from build123d import *

# Parameters (mm, degrees)
F0_R     = 1.55
F0_R_2   = 2.05
F0_R_3   = 11
F1_DEPTH = 4


with BuildPart() as f1:
    # F0 (on Front) → F1 (new body)
    with BuildSketch(Plane.XZ):
        with BuildLine():
            Line((-12.9276869952, -14.7702103927), (49.2744245402, -25.0594563055))
            ThreePointArc((49.2744245402, -25.0594563055), (61.2632923167, -19.4743843221), (57.2253318853, -6.8799071524))
            Line((57.2253318853, -6.8799071524), (-12.5790872929, 34.7723583687))
            Line((-12.5790872929, 34.7723583687), (-35.6180453168, 48.5196942571))
            ThreePointArc((-35.6180453168, 48.5196942571), (-39.3883061053, 49.0778177624), (-42.4565310048, 46.8167639757))
            Line((-42.4565310048, 46.8167639757), (-44.283169795, 43.8016410413))
            Line((-44.283169795, 43.8016410413), (-68.4894634868, 3.7363676474))
            ThreePointArc((-68.4894634868, 3.7363676474), (-69.1796280017, 0.6014549382), (-67.8214663387, -2.3070501159))
            Line((-67.8214663387, -2.3070501159), (-54.0816127895, -16.6578253643))
            ThreePointArc((-54.0816127895, -16.6578253643), (-52.4335683043, -17.7983223484), (-50.4700412586, -18.200000748))
            Line((-50.4700412586, -18.200000748), (-21.8383905306, -18.200000748))
            ThreePointArc((-21.8383905306, -18.200000748), (-20.3097897038, -17.960607801), (-18.9275633798, -17.265352553))
            Line((-18.9275633798, -17.265352553), (-16.6545073746, -15.6378247392))
            ThreePointArc((-16.6545073746, -15.6378247392), (-14.877378135, -14.8333994398), (-12.9276869952, -14.7702103927))
        make_face()
        with BuildLine():
            ThreePointArc((-46.4896173713, 5.2461908635), (-45.1396173713, 6.5961908635), (-43.7896173713, 5.2461908635))
            Line((-43.7896173713, 5.2461908635), (-43.7896173713, -12.7538091365))
            ThreePointArc((-43.7896173713, -12.7538091365), (-45.1396173713, -14.1038091365), (-46.4896173713, -12.7538091365))
            Line((-46.4896173713, -12.7538091365), (-46.4896173713, 5.2461908635))
        make_face(mode=Mode.SUBTRACT)
        with BuildLine():
            Line((-41.1896173713, -13.2911801338), (-41.1896173713, 5.2461908635))
            ThreePointArc((-41.1896173713, 5.2461908635), (-38.1396173713, 8.2961908635), (-35.0896173713, 5.2461908635))
            Line((-35.0896173713, 5.2461908635), (-35.0896173713, -13.2911801338))
            ThreePointArc((-35.0896173713, -13.2911801338), (-38.1396173713, -16.3411801338), (-41.1896173713, -13.2911801338))
        make_face(mode=Mode.SUBTRACT)
        with Locations((-58.3313559954, 8.044780269)):
            Circle(F0_R, mode=Mode.SUBTRACT)
        with BuildLine():
            Line((-32.4896173713, -12.7538091365), (-32.4896173713, 5.2461908635))
            ThreePointArc((-32.4896173713, 5.2461908635), (-31.1396173713, 6.5961908635), (-29.7896173713, 5.2461908635))
            Line((-29.7896173713, 5.2461908635), (-29.7896173713, -12.7538091365))
            ThreePointArc((-29.7896173713, -12.7538091365), (-31.1396173713, -14.1038091365), (-32.4896173713, -12.7538091365))
        make_face(mode=Mode.SUBTRACT)
        with Locations((52.1012294587, -15.4673150455)):
            Circle(F0_R_2, mode=Mode.SUBTRACT)
        with Locations((-38.1396173713, 25.2461908635)):
            Circle(F0_R_3, mode=Mode.SUBTRACT)
        with Locations((-19.0286114888, 17.7422984931)):
            Circle(F0_R, mode=Mode.SUBTRACT)
        with Locations((-37.8051390947, 41.9450122359)):
            Circle(F0_R, mode=Mode.SUBTRACT)
    extrude(amount=F1_DEPTH)


solid = f1.part
Design review of the part built by this model. Coordinates are the model's own, in mm. A direction names the side the tool comes from. Round coordinates to 2 decimals unless told otherwise and drop trailing zeros. Write each loop counter-clockwise with the first axis right and the second up, starting at its lowest first coordinate (ties: lowest second). Pieces come first, ordered by that corner, then holes. Notation, with made-up numbers: (50, 10) - (78, 10) arc R27 ccw to (78, 47) - close; hole circle Ø2 at (52, -29.5). An arc over 180 degrees is marked (long way). Return JSON: item names as keys, results as strings. Group by question number.
Item 1: For probe 1 along X at (y, z) = (-2.6, -11); probe 2 along Z at (x, y) = (-31, -2.05); probe 3 along X at (y, z) = (-1.95, -6.5), list the stretches that pass through material, from the lowest coordinate up. Write a range as [from, to].
Item 2: The part is to be moulded in two halves that separate along Z. For faces 1 (the face through (-14.9, -1.97, -14.84)), 2 (the face through (-59.88, -1.97, 8.11)), 3 (the face through (-4, -4, 4)), say which applies: pulls with the +Z half, pulls with the -Z half, needs draft (parallel to the pull), parting line crosses it, or undercut.
Item 3: We need section A-A on z = 2. Write out the cut boundary in (x, y), and give its area (3 significant figures).
Item 4: Machinability: for faces 4 (the face through (-69.184, -1.972, 0.647)), 5 (the face through (-20.331, -1.972, -17.967)), 6 (the face through (-32.49, -2, -4)), which of the approach directions +Z, -Z, +X, -X, +Y, -Y give a long, thin tool a straight path to every point of the face, cutting with its end or side? Answer none if there is none.
Item 5: We need section C-C on z = 32.5. Write out the cut boundary in (x, y), and give its area (3 significant figures).
Item 6: We need section D-D on x = 36. Write out the cut boundary in (y, z), and give its area (3 significant figures).
Item 7: We need section B-B on y = -2.5. Give the number of separate pieces and of enclosed holes in the cut face, and give its area (3 significant figures).
Item 8: Insertion check: P1, Ø5, axis at x = -58.33, z = 8.04, coming from the -Y side; P2, Ø2, axis at x = 14.5, y = -0.5, coming from the +Z side; P3, Ø1, axis at x = 32.5, y = -0.5, coming from the -Z side; P4, Ø1.2, axis at y = -3, z = -0.5, coming from the -X side. Each pin has a flat end and moves straight along its axis. Give the tip position at first contact, or say it passes through.
Model answer:
{
 "1": {"probe 1": "x = [-59.5, -46.49], [-43.79, -41.19], [-35.09, -32.49], [-29.79, 61.05]", "probe 2": "z = [-18.2, -14.1], [6.59, 16.88], [33.61, 45.76]", "probe 3": "x = [-63.81, -46.49], [-43.79, -41.19], [-35.09, -32.49], [-29.79, 56.59]"},
 "2": {"face 1": "pulls with the -Z half", "face 2": "undercut", "face 3": "needs draft"},
 "3": {"outline": "(-69.14, -4) - (-46.49, -4) - (-46.49, 0) - (-69.14, 0) - close; (-43.79, -4) - (-41.19, -4) - (-41.19, 0) - (-43.79, 0) - close; (-35.09, -4) - (-32.49, -4) - (-32.49, 0) - (-35.09, 0) - close; (-29.79, -4) - (42.34, -4) - (42.34, 0) - (-29.79, 0) - close", "area": "400 mm²"},
 "4": {"face 4": "-X, +Y, -Y", "face 5": "-Z, +Y, -Y", "face 6": "+Y, -Y"},
 "5": {"outline": "(-51.11, -4) - (-46.41, -4) - (-46.41, 0) - (-51.11, 0) - close; (-29.87, -4) - (-8.77, -4) - (-8.77, 0) - (-29.87, 0) - close", "area": "103 mm²"},
 "6": {"outline": "(-4, -22.86) - (0, -22.86) - (0, 5.79) - (-4, 5.79) - close", "area": "115 mm²"},
 "7": {"separate pieces": "1", "enclosed holes": "8", "area": "4,620 mm²"},
 "8": {"P1": "stops at y = -4", "P2": "stops at z = 19.21", "P3": "stops at z = -22.37", "P4": "stops at x = -69.1"}
}
